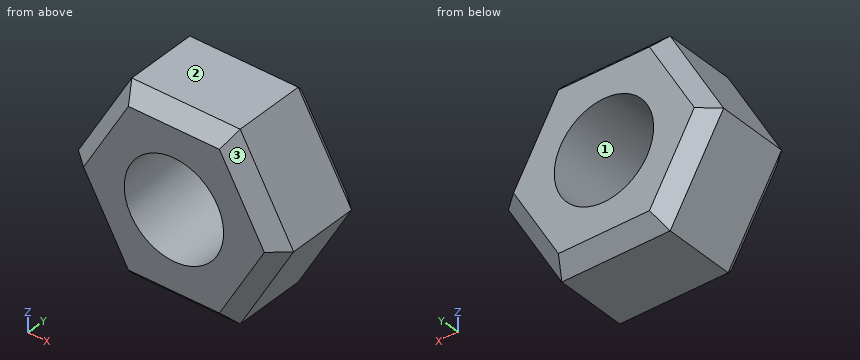
Autodesk Inventor part; units mm, degrees
ref_plane "YZ Plane" through (0, 0, 0) normal (1, 0, 0) x (0, 1, 0)
ref_plane "XZ Plane" through (0, 0, 0) normal (0, 1, 0) x (-1, 0, 0)
ref_plane "XY Plane" through (0, 0, 0) normal (0, 0, 1) x (1, 0, 0)
sketch "草图1" plane through (0, 0, 0) normal (0, 1, 0) x (-1, 0, 0)
  line L0 (0, 0) -> (7.2, 0)
  line L1 (7.2, 0) -> (3.6254, -6.25)
  line L2 (3.6254, -6.25) -> (0, -6.25)
  line L3 (7.2, 0) -> (3.6254, 6.25)
  line L4 (3.6254, 6.25) -> (0, 6.25)
  line L5 (0, 0) -> (0, -6.25)
  line L6 (-7.2, 0) -> (-3.6254, -6.25)
  line L7 (-3.6254, -6.25) -> (0, -6.25)
  line L8 (-7.2, 0) -> (-3.6254, 6.25)
  line L9 (-3.6254, 6.25) -> (0, 6.25)
  dimension "d2" = 14.4
  dimension "d3" = 12.5
extrude "拉伸1" add sketch "草图1" along normal blind 6.8
sketch "草图2" plane through (0, 6.8, 0) normal (0, 1, 0) x (1, 0, 0)
  circle A0 centre (0, 0) radius 6.25
  dimension "d6" = 12.5
hole "孔1" at (0, 6.8, 0) direction (0, -1, 0) diameter 6.647 end through all
chamfer "倒角3" distance 1 angle 45 12 edges at (0, 6.8, 6.25) (5.4127, 6.8, 3.125) (5.4127, 6.8, -3.125) (0, 6.8, -6.25) (-5.4127, 6.8, -3.125) (-5.4127, 6.8, 3.125) (5.4127, 0, 3.125) (5.4127, 0, -3.125) (0, 0, -6.25) (-5.4127, 0, -3.125) (-5.4127, 0, 3.125) (0, 0, 6.25)
properties part number "6-luomu" material "不锈钢"
CAD build for the part. Positions are in the model's coordinates, mm. Face numbers are marked on the shaded views. Coordinates: 2 decimals unless noted, no trailing zeros. Write each loop counter-clockwise with the first axis right and the second up, starting at its lowest first coordinate (ties: lowest second). Pieces come first, ordered by that corner, then holes. Notation, with made-up numbers: (-40, -15) -> (-36, -15) arc R12 cw to (-36, 1) -> close; hole circle Ø5 at (40, -17.75). An arc over 180 degrees is marked (long way). Use CSV: the item, a comma, the result in double quotes. Start each with the question number.
Item 1: Drop flat-ended pins along their axis: P1, Ø1, axis at y = 2, z = -3, coming from the -X side; P2, Ø1, axis at y = 4.5, z = 4.5, coming from the -X side; P3, Ø1, axis at x = -5.5, y = 1, coming from the +Z side. Give the stop position or say it passes through.
Item 2: Band-saw the part on C-C, the plane y = 4. Write the cut outline in (x, z).
Item 3: Band-saw the part on B-B, the plane z = -3. Write the cut outline in (x, y), plus the area to 3 significant figures.
Item 4: Wall check: probe 1 along Z at (x, y) = (0, 5); probe 2 along Z at (x, y) = (2.5, 6.5); probe 3 along X at (y, z) = (2, 2.25). Give the ranges that are in metal, low to high.
Item 5: Band-saw the part on D-D, the plane z = 3.75. Write the cut outline in (x, y).
Item 6: Band-saw the part on A-A, the plane x = 0. Write the cut outline in (y, z).
Item 7: Two-plate mould, pull along X, no slides. Class the marked faces 1, 2 and 3: +X half, -X half, draft (parallel to the pull), parting line (faces both ways), or undercut.
Response values:
1,P1,"stops at x = -5.77"
1,P2,"stops at x = -4.91"
1,P3,"stops at z = 3.85"
2,outline,"(-7.2, 0) -> (-3.63, -6.25) -> (3.63, -6.25) -> (7.2, 0) -> (3.63, 6.25) -> (-3.63, 6.25) -> close; hole circle Ø6.65 at (0, 0)"
3,outline,"(-5.48, 1) -> (-4.33, 0) -> (-1.43, 0) -> (-1.43, 6.8) -> (-4.33, 6.8) -> (-5.48, 5.8) -> close; (1.43, 0) -> (4.33, 0) -> (5.48, 1) -> (5.48, 5.8) -> (4.33, 6.8) -> (1.43, 6.8) -> close"
3,area,"52.8 mm2"
4,probe 1,"z = -6.25 to -3.32, 3.32 to 6.25"
4,probe 2,"z = -5.55 to -2.19, 2.19 to 5.55"
4,probe 3,"x = -5.91 to -2.45, 2.45 to 5.91"
5,outline,"(-5.06, 1) -> (-3.9, 0) -> (3.9, 0) -> (5.06, 1) -> (5.06, 5.8) -> (3.9, 6.8) -> (-3.9, 6.8) -> (-5.06, 5.8) -> close"
6,outline,"(0, -5.25) -> (1, -6.25) -> (5.8, -6.25) -> (6.8, -5.25) -> (6.8, -3.32) -> (0, -3.32) -> close; (0, 3.32) -> (6.8, 3.32) -> (6.8, 5.25) -> (5.8, 6.25) -> (1, 6.25) -> (0, 5.25) -> close"
7,face 1,"undercut"
7,face 2,"draft"
7,face 3,"+X half"
